```python
from build123d import *

# Parameters (mm, degrees)
EXTRUDE_1_DEPTH = 500


with BuildPart() as part:
    # 草图9 → 拉伸1 (new body, symmetric)
    with BuildSketch(Plane.XY):
        with BuildLine():
            Line((-1, 18), (-0.997378521, 4))
            ThreePointArc((-0.997378521, 4), (-1.29027174, 3.292893219), (-1.997378521, 3))
            Line((-1.997378521, 3), (-9.5, 3))
            ThreePointArc((-9.5, 3), (-10.207106781, 3.292893219), (-10.5, 4))
            Line((-10.5, 4), (-10.5, 18))
            Line((-10.5, 18), (-10.962126781, 19.848507125))
            ThreePointArc((-10.962126781, 19.848507125), (-11.033072839, 19.957641088), (-11.156155281, 20))
            Line((-11.156155281, 20), (-12.8, 20))
            ThreePointArc((-12.8, 20), (-12.941421356, 19.941421356), (-13, 19.8))
            Line((-13, 19.8), (-13, 1))
            ThreePointArc((-13, 1), (-12.707106781, 0.292893219), (-12, 0))
            Line((-12, 0), (-3.712080642, 0))
            Line((-3.712080642, 0), (-4.1, -2.2))
            Line((-4.1, -2.2), (-4.395740138, -2.712236945))
            Line((-4.395740138, -2.712236945), (-3.363574657, -4.5))
            ThreePointArc((-3.363574657, -4.5), (-2.680561955, -4.683012702), (-2.497549254, -4))
            Line((-2.497549254, -4), (-3.190369577, -2.8))
            Line((-3.190369577, -2.8), (-2.769508091, -0.413175911))
            ThreePointArc((-2.769508091, -0.413175911), (-2.59849802, -0.116977778), (-2.277104215, 0))
            Line((-2.277104215, 0), (2.277104215, 0))
            ThreePointArc((2.277104215, 0), (2.59849802, -0.116977778), (2.769508091, -0.413175911))
            Line((2.769508091, -0.413175911), (3.190369577, -2.8))
            Line((3.190369577, -2.8), (2.497549254, -4))
            ThreePointArc((2.497549254, -4), (2.680561955, -4.683012702), (3.363574657, -4.5))
            Line((3.363574657, -4.5), (4.395740138, -2.712236945))
            Line((4.395740138, -2.712236945), (4.1, -2.2))
            Line((4.1, -2.2), (3.712080642, 0))
            Line((3.712080642, 0), (12, 0))
            ThreePointArc((12, 0), (12.707106781, 0.292893219), (13, 1))
            Line((13, 1), (13, 19.8))
            ThreePointArc((13, 19.8), (12.941421356, 19.941421356), (12.8, 20))
            Line((12.8, 20), (11.158776943, 20))
            ThreePointArc((11.158776943, 20), (11.035799699, 19.957723167), (10.964813339, 19.848765973))
            Line((10.964813339, 19.848765973), (10.5, 18))
            Line((10.5, 18), (10.5, 4))
            ThreePointArc((10.5, 4), (10.207106781, 3.292893219), (9.5, 3))
            Line((9.5, 3), (2, 3))
            ThreePointArc((2, 3), (1.292893219, 3.292893219), (1, 4))
            Line((1, 4), (1, 18))
            Line((1, 18), (0.537873219, 19.848507125))
            ThreePointArc((0.537873219, 19.848507125), (0.466927161, 19.957641088), (0.343844719, 20))
            Line((0.343844719, 20), (-0.34122324, 20))
            ThreePointArc((-0.34122324, 20), (-0.464305682, 19.957641088), (-0.53525174, 19.848507125))
            Line((-0.53525174, 19.848507125), (-1, 18))
        make_face()
    extrude(amount=EXTRUDE_1_DEPTH, both=True)


solid = part.part
```
The model under review builds one solid part; all positions refer to its coordinate system, in mm. Coordinates: 2 decimals unless noted, no trailing zeros. Order: outer loops, then holes, each group sorted by start corner. A loop starts at its lowest first (then second) coordinate and runs counter-clockwise, first axis right, second up. Notation, with made-up numbers: (-17, 48.25) -> (12, 48.25) arc R14 ccw to (12, 57.25) -> close; hole circle Ø5 at (86, -25). An arc over 180 degrees is marked (long way). Answer in a Markdown table with one row per item. Add a question column.
Item 1: We need section A-A on y = 13.5. Write out the cut boundary in (x, z), plus the area to 3 significant figures.
Item 2: To check wall thickness, follow probe 1 along X at (y, z) = (11.25, 144.5); probe 2 along Y at (x, z) = (2.5, 42.5); probe 3 along X at (y, z) = (-1, -264). State the ranges of each line that lie inside material, in increasing order.
Item 3: Clearance check with flat-ended pins moving along their axes: pin 1 (4 mm diameter, centred on x = -6, z = 146.5, fed in from +Y); pin 2 (6 mm diameter, centred on x = 7, z = -24, fed in from -Y); pin 3 (1.4 mm diameter, centred on x = -0.5, z = -87.5, fed in from -Y); pin 4 (10 mm diameter, centred on x = 7.5, y = 6.5, fed in from +Z). State where each tip first meets the part, or that it passes through.
Item 4: Mouldability with a two-part tool opening along X and no side actions: class faces 1 (the flat face through (13, 10, 7)), 2 (the flat face through (0, 6, -500)), 3 (the flat face through (-13, 11, 7)) as +X half, -X half, draft (parallel to the pull), parting line (faces both ways), or undercut.
Final values:
| question | item | result |
|---|---|---|
| 1 | outline | (-13, -500) -> (-10.5, -500) -> (-10.5, 500) -> (-13, 500) -> close; (-1, -500) -> (1, -500) -> (1, 500) -> (-1, 500) -> close; (10.5, -500) -> (13, -500) -> (13, 500) -> (10.5, 500) -> close |
| 1 | area | 7,000 mm2 |
| 2 | probe 1 | x = -13 to -10.5, -1 to 1, 10.5 to 13 |
| 2 | probe 2 | y = -4.5 to -4, -0.05 to 3 |
| 2 | probe 3 | x = -3.89 to -2.87, 2.87 to 3.89 |
| 3 | pin 1 | stops at y = 3 |
| 3 | pin 2 | stops at y = -3.4 |
| 3 | pin 3 | stops at y = 0 |
| 3 | pin 4 | stops at z = 500 |
| 4 | face 1 | +X half |
| 4 | face 2 | draft |
| 4 | face 3 | -X half |
